```python
from build123d import *

# Parameters (mm, degrees)
SKETCH_W       = 20
SKETCH_H       = 20
PAD_DEPTH      = 40
SKETCH001_R    = 1.65
HOLE_DEPTH     = 8
HOLE_TIPS_R    = 1.65
SKETCH002_R    = 1.65
HOLE001_DEPTH  = 8
HOLE001_TIPS_R = 1.65


with BuildPart() as part:
    # Sketch → Pad (new body)
    with BuildSketch(Plane.XY):
        with Locations((-75, 10)):
            Rectangle(SKETCH_W, SKETCH_H)
    extrude(amount=PAD_DEPTH)

    # Sketch001 (on Face1 of Pad) → Hole (cut)
    with BuildSketch(Plane.XZ):
        with Locations((-75, 30)):
            Circle(SKETCH001_R)
        with Locations((-75, 10)):
            Circle(SKETCH001_R)
    extrude(amount=-HOLE_DEPTH, mode=Mode.SUBTRACT)

    # Hole tips → Hole tip 1 section 0
    with BuildSketch(Plane.XZ.offset(-8), mode=Mode.PRIVATE) as hole_tip_1_s0:
        with Locations((-75, 30)):
            Circle(HOLE_TIPS_R)
    loft([hole_tip_1_s0.sketch, Vertex(-75, 8.99142, 30)], mode=Mode.SUBTRACT)

    # Hole tips → Hole tip 2 section 0
    with BuildSketch(Plane.XZ.offset(-8), mode=Mode.PRIVATE) as hole_tip_2_s0:
        with Locations((-75, 10)):
            Circle(HOLE_TIPS_R)
    loft([hole_tip_2_s0.sketch, Vertex(-75, 8.99142, 10)], mode=Mode.SUBTRACT)

    # Sketch002 (on Face4 of Hole) → Hole001 (cut)
    with BuildSketch(Plane.XY.offset(40)):
        with Locations((-70, 10)):
            Circle(SKETCH002_R)
    extrude(amount=-HOLE001_DEPTH, mode=Mode.SUBTRACT)

    # Hole001 tips → Hole001 tip 1 section 0
    with BuildSketch(Plane.XY.offset(32), mode=Mode.PRIVATE) as hole001_tip_1_s0:
        with Locations((-70, 10)):
            Circle(HOLE001_TIPS_R)
    loft([hole001_tip_1_s0.sketch, Vertex(-70, 10, 31.00858)], mode=Mode.SUBTRACT)


solid = part.part
```
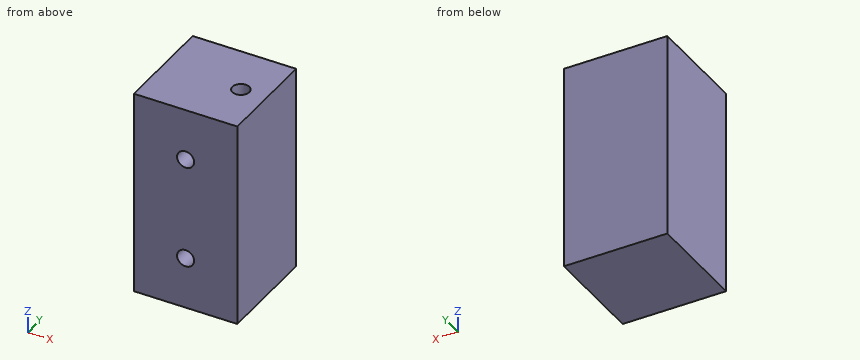
The model under review builds one solid part; all positions refer to its coordinate system, in mm. Coordinates: 2 decimals unless noted, no trailing zeros. Write each loop counter-clockwise with the first axis right and the second up, starting at its lowest first coordinate (ties: lowest second). Pieces come first, ordered by that corner, then holes. Notation, with made-up numbers: (39.25, 77.5) - (63.25, 77.5) arc R33 cw to (63.25, 107.5) - close; hole circle Ø6 at (3, 25.5). An arc over 180 degrees is marked (long way). Write item = value, one per line.
(1) Consider section A-A, the plane y = 2.5. Give the boundary of the cut face in (x, z), then the cut area to 3 significant figures.
Result sheet:
outline = (-85, 0) - (-65, 0) - (-65, 40) - (-85, 40) - close; hole circle Ø3.3 at (-75, 10); hole circle Ø3.3 at (-75, 30)
area = 783 mm^2
(2) For line 1 (Z direction, x = -75, y = 4.75); line 2 (Y direction, x = -70, z = 37.25), list the stretches that pass through material, from the lowest coordinate up. Write a range as [from, to].
Result sheet:
line_1 = [0, 8.35], [11.65, 28.35], [31.65, 40]
line_2 = [0, 8.35], [11.65, 20]
(3) For P1, Ø2.5, axis at x = -70, y = 10, coming from the +Z side, flat-tipped, find the tip position at first contact; note if it passes through.
Result sheet:
P1 = 31.76
